Model file for the job. Use its own axes, mm. A direction names the side the tool comes from. Round coordinates to 2 decimals unless told otherwise and drop trailing zeros. Loops run counter-clockwise (first coordinate to the right, second up) from the corner with the lowest first, then second, coordinate; pieces in that order, holes last. Notation, with made-up numbers: (85, 71) -> (95, 71) arc R10 cw to (95, 87) -> close; hole circle Ø5 at (3.25, 21). An arc over 180 degrees is marked (long way). Use a Markdown table: item, result. Add a question column.
```python
from build123d import *

# Parameters (mm, degrees)
SKETCH1_W           = 45
SKETCH1_H           = 150
BOSS_EXTRUDE1_DEPTH = 0.5
SKETCH2_R           = 2.25
CUT_EXTRUDE1_DEPTH  = 10.5
HEM1_START          = -75
HEM1_DEPTH          = 150
HEM1_2_DEPTH        = 150


# Read off the part's stored shape, not the designer's step: Hem1
with BuildPart() as part:
    # Sketch1 → Boss-Extrude1 (new body)
    with BuildSketch(Plane(origin=(0, 0, 0), x_dir=(1, 0, 0), z_dir=(0, 1, 0))):
        Rectangle(SKETCH1_W, SKETCH1_H)
    extrude(amount=BOSS_EXTRUDE1_DEPTH)

    # Sketch2 → Cut-Extrude1 (cut)
    with BuildSketch(Plane(origin=(0, 0.5, 0), x_dir=(1, 0, 0), z_dir=(0, 1, 0))):
        with Locations(Location((0, 52.5, 0), (0, 0, 270))):
            Circle(SKETCH2_R)
        with Locations(Location((0, 17.5, 0), (0, 0, 270))):
            Circle(SKETCH2_R)
        with Locations(Location((0, -17.5, 0), (0, 0, 270))):
            Circle(SKETCH2_R)
        with Locations(Location((0, -52.5, 0), (0, 0, 270))):
            Circle(SKETCH2_R)
    extrude(amount=-CUT_EXTRUDE1_DEPTH, mode=Mode.SUBTRACT)

    # Hem1 outline → Hem1 (cut)
    with BuildSketch(Plane.XY.offset(HEM1_START)):
        with BuildLine():
            ThreePointArc((21.95, 0.5), (22.320809924, 0.35620192), (22.497722558, 0))
            Line((22.497722558, 0), (22.5, 0))
            Line((22.5, 0), (22.5, 0.5))
            Line((22.5, 0.5), (21.95, 0.5))
        make_face()
        with BuildLine():
            ThreePointArc((-22.497722558, 0), (-22.320809924, 0.35620192), (-21.95, 0.5))
            Line((-21.95, 0.5), (-22.5, 0.5))
            Line((-22.5, 0.5), (-22.5, 0))
            Line((-22.5, 0), (-22.497722558, 0))
        make_face()
    extrude(amount=HEM1_DEPTH, mode=Mode.SUBTRACT)

    # Hem1 2 outline → Hem1 2 (add)
    with BuildSketch(Plane.XY.offset(HEM1_START)):
        with BuildLine():
            Line((12.5, -0.1), (12.5, -0.6))
            Line((12.5, -0.6), (21.95, -0.6))
            ThreePointArc((21.95, -0.6), (22.35620192, -0.420809924), (22.497722558, 0))
            Line((22.497722558, 0), (21.95, 0))
            ThreePointArc((21.95, 0), (22, -0.05), (21.95, -0.1))
            Line((21.95, -0.1), (12.5, -0.1))
        make_face()
        with BuildLine():
            ThreePointArc((-21.95, -0.1), (-22, -0.05), (-21.95, 0))
            Line((-21.95, 0), (-22.497722558, 0))
            ThreePointArc((-22.497722558, 0), (-22.35620192, -0.420809924), (-21.95, -0.6))
            Line((-21.95, -0.6), (-12.5, -0.6))
            Line((-12.5, -0.6), (-12.5, -0.1))
            Line((-12.5, -0.1), (-21.95, -0.1))
        make_face()
    extrude(amount=HEM1_2_DEPTH)


solid = part.part
```
1) Cut at C-C on x = 0. Write the cut outline in (y, z).
2) Cut at B-B on z = 52.5. Write the cut outline in (x, y), and give its area (3 significant figures).
3) Cut at A-A on x = -16. Write the cut outline in (y, z), and give its area (3 significant figures).
4) Tool access for faces 1 (the face through (0, 0, -1)), 2 (the face through (0.099, 0.254, 50.252)): list every direction of +Z, -Z, +X, -X, +Y, -Y with a clear straight run to the whole face (end or side of a thin tool).
5) Pin check, flat tips, straight feed: pin 1 Ø0.6 at (y, z) = (-0.5, 21.5) entering from -X; pin 2 Ø2.5 at (x, z) = (0, 17.5) entering from -Y; pin 3 Ø0.6 at (y, z) = (-0.5, 5.5) entering from +X. Stop position of each tip, or through.
6) Wall check: probe 1 along X at (y, z) = (-0.05, 67.5); probe 2 along Z at (x, y) = (-0.5, 0.3); probe 3 along X at (y, z) = (0.25, -52.5). Give the ranges that are in metal, low to high. Write a range as from..to.
7) Cut at D-D on z = -10.5. Write the cut outline in (x, y).
8) Pull direction X, two halves, no side cores. Call faces 3 (the face through (0, 0.5, -1)), 4 (the face through (0.676, 0.254, 19.646)): +X half, -X half, draft (parallel to the pull), parting line (faces both ways), or undercut.
Established:
| question | item | result |
|---|---|---|
| 1 | outline | (0, -75) -> (0.5, -75) -> (0.5, -54.75) -> (0, -54.75) -> close; (0, -50.25) -> (0.5, -50.25) -> (0.5, -19.75) -> (0, -19.75) -> close; (0, -15.25) -> (0.5, -15.25) -> (0.5, 15.25) -> (0, 15.25) -> close; (0, 19.75) -> (0.5, 19.75) -> (0.5, 50.25) -> (0, 50.25) -> close; (0, 54.75) -> (0.5, 54.75) -> (0.5, 75) -> (0, 75) -> close |
| 2 | outline | (-21.95, -0.6) -> (-12.5, -0.6) -> (-12.5, -0.1) -> (-21.95, -0.1) arc R0.05 cw to (-21.95, 0) -> (-2.25, 0) -> (-2.25, 0.5) -> (-21.95, 0.5) arc R0.55 ccw to start; (2.25, 0) -> (21.95, 0) arc R0.05 cw to (21.95, -0.1) -> (12.5, -0.1) -> (12.5, -0.6) -> (21.95, -0.6) arc R0.55 ccw to (21.95, 0.5) -> (2.25, 0.5) -> close |
| 2 | area | 30.1 mm^2 |
| 3 | outline | (-0.6, -75) -> (-0.1, -75) -> (-0.1, 75) -> (-0.6, 75) -> close; (0, -75) -> (0.5, -75) -> (0.5, 75) -> (0, 75) -> close |
| 3 | area | 150 mm^2 |
| 4 | face 1 | +Z, -Z |
| 4 | face 2 | +Y, -Y |
| 5 | pin 1 | stops at x = -22.48 |
| 5 | pin 2 | passes through |
| 5 | pin 3 | stops at x = 22.48 |
| 6 | probe 1 | x = -22.5..-22, 22..22.5 |
| 6 | probe 2 | z = -75..-54.69, -50.31..-19.69, -15.31..15.31, 19.69..50.31, 54.69..75 |
| 6 | probe 3 | x = -22.41..-2.25, 2.25..22.41 |
| 7 | outline | (-21.95, -0.6) -> (-12.5, -0.6) -> (-12.5, -0.1) -> (-21.95, -0.1) arc R0.05 cw to (-21.95, 0) -> (21.95, 0) arc R0.05 cw to (21.95, -0.1) -> (12.5, -0.1) -> (12.5, -0.6) -> (21.95, -0.6) arc R0.55 ccw to (21.95, 0.5) -> (-21.95, 0.5) arc R0.55 ccw to start |
| 8 | face 3 | draft |
| 8 | face 4 | undercut |
